The figure shows three views and two pictorial views of one solid part (mm, origin at its lowest corner). Answer the questions. A direction names the side the tool comes from. Give positions to 0.01 mm unless a question says otherwise; leave off trailing zeros. Write each loop counter-clockwise with the first axis right and the second up, starting at its lowest first coordinate (ties: lowest second). Pieces come first, ordered by that corner, then holes. Notation, with made-up numbers: M 12,-33.5 L 46,-33.5 A28 ccw 46,5.5 Z; hole C 61.5,16.25 d9. An arc over 180 degrees is marked long. Return JSON: item names as keys, results as strings.
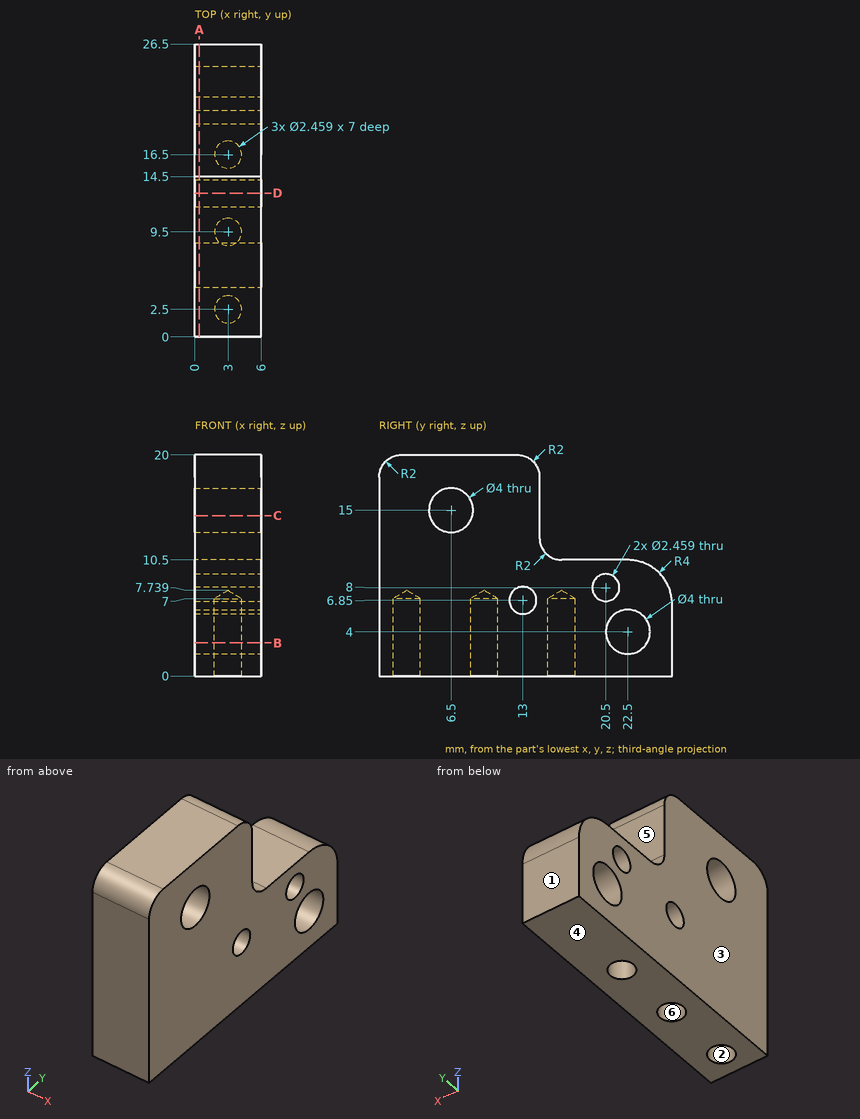
Item 1: A cutting plane is placed at A-A, the plane x = 0.4. Write down the section's boundary in (y, z), plus the area to 3 significant figures.
Geometry results:
{"outline": "M 0,0 L 26.5,0 L 26.5,6.5 A4 ccw 22.5,10.5 L 16.5,10.5 A2 cw 14.5,12.5 L 14.5,18 A2 ccw 12.5,20 L 2,20 A2 ccw 0,18 Z; hole C 6.5,15 d4; hole C 13,6.85 d2.46; hole C 20.5,8 d2.46; hole C 22.5,4 d4", "area": "377 mm2"}
Item 2: Find the intervals of material crossed by line 1 (Y direction, x = 2.9, z = 15); line 2 (Z direction, x = 3.15, y = 6.5); line 3 (Y direction, x = 4.05, z = 6.5), in increasing order.
Geometry results:
{"line 1": "y = 0 to 4.5, 8.5 to 14.5", "line 2": "z = 0 to 13, 17 to 20", "line 3": "y = 0 to 1.86, 3.14 to 8.86, 10.14 to 11.82, 14.18 to 15.86, 17.14 to 26.5"}
Item 3: Determine the mould class of the marked faces 1, 2 and 3 for opening direction X: +X half, -X half, draft (parallel to the pull), parting line (faces both ways), or undercut.
Geometry results:
{"face 1": "draft", "face 2": "undercut", "face 3": "-X half"}
Item 4: A cutting plane is placed at D-D, the plane y = 13. Write down the section's boundary in (x, z).
Geometry results:
{"outline": "M 0,0 L 6,0 L 6,5.62 L 0,5.62 Z; M 0,8.08 L 6,8.08 L 6,19.94 L 0,19.94 Z"}
Item 5: Which of the six approach directions +Z, -Z, +X, -X, +Y, -Y give full straight-line access (tool end or side, diameter ignored) to the marked faces 4, 5 and 6?
Geometry results:
{"face 4": "-Z, +X, -X, +Y, -Y", "face 5": "+Z, +X, -X, +Y", "face 6": "-Z"}
Item 6: Given pin 1 Ø1.5 at (x, y) = (3, 9.5) entering from -Z; pin 2 Ø2 at (x, z) = (3, 8) entering from +Y; pin 3 Ø3 at (x, z) = (4, 16.5) entering from +Y, each flat-ended and moving along its own axis, determine where each tip first touches the part or whether it passes through.
Geometry results:
{"pin 1": "stops at z = 7.29", "pin 2": "stops at y = 26.47", "pin 3": "stops at y = 14.5"}
Item 7: A cutting plane is placed at C-C, the plane z = 14.5. Write down the section's boundary in (x, y).
Geometry results:
{"outline": "M 0,0 L 6,0 L 6,4.56 L 0,4.56 Z; M 0,8.44 L 6,8.44 L 6,14.5 L 0,14.5 Z"}
Item 8: A cutting plane is placed at B-B, the plane z = 3. Write down the section's boundary in (x, y), plus the area to 3 significant figures.
Geometry results:
{"outline": "M 0,0 L 6,0 L 6,20.77 L 0,20.77 Z; M 0,24.23 L 6,24.23 L 6,26.5 L 0,26.5 Z; hole C 3,2.5 d2.46; hole C 3,9.5 d2.46; hole C 3,16.5 d2.46", "area": "124 mm2"}
